Verification items for the finished model (mm, model axes). A direction names the side the tool comes from. Coordinates: 2 decimals unless noted, no trailing zeros. Order: outer loops, then holes, each group sorted by start corner. A loop starts at its lowest first (then second) coordinate and runs counter-clockwise, first axis right, second up.
Q1. Draft check along Z on faces 1 (the flat face through (7, -1, 21)), 2 (the flat face through (3, -6, 34)), 3 (the flat face through (3, -2, 27)). Enter one of: pulls with the +Z half, pulls with the -Z half, needs draft (parallel to the pull), parting line crosses it, or undercut.
Q2. Set-up check for faces 4 (the flat face through (3, -4.8, 3)), 5 (the flat face through (1.9, -2, 11.3)), 6 (the flat face through (3, -10.5, 27)): record each of +Z, -Z, +X, -X, +Y, -Y from which the full face is reachable in a straight line by a thin tool's end or side.
Q3. Thickness scan on line 1 (Z direction, x = 6, y = -8.75); line 2 (Y direction, x = 2.5, z = 25); line 3 (Y direction, x = 1, z = 5.5). Record the ranges inside material, lowest first.
Q4. Cross-section at A-A, the plane z = 10. Record the boundary of the cut face in (x, y), and give its area (3 significant figures).
Q5. Cross-section at D-D, the plane x = 6.25. Record the boundary of the cut face in (y, z), and give its area (3 significant figures).
Q6. Cross-section at B-B, the plane x = 3.5. Count the separate pieces of the cut face and the enclosed holes in it, and give its area (3 significant figures).
Q7. Depth check by flat-ended pin: P1, Ø0.7, axis at x = 5, z = 17, coming from the -Y side; P2, Ø0.7, axis at x = 3.5, y = -3, coming from the -Z side; P3, Ø2, axis at x = 6, z = 6, coming from the -Y side. Enter the tip coordinate at first touch or a pass-through.
Q8. Cross-section at C-C, the plane y = -8.75. Record the boundary of the cut face in (x, z).
from build123d import *

# Parameters (mm, degrees)
F0_W     = 7
F0_H     = 20
F0_R     = 1.75
F1_DEPTH = 2
F3_DEPTH = 2.8
F4_R     = 0.5
F5_R     = 0.5
F6_W     = 8.5
F6_H     = 8.979
F7_DEPTH = 7
F8_R     = 2.5
F9_R     = 1


with BuildPart() as f1:
    # F0 (on Front) → F1 (new body)
    with BuildSketch(Plane.XZ):
        with Locations((3.5, 10)):
            Rectangle(F0_W, F0_H)
        with Locations((3.5, 10)):
            Circle(F0_R, mode=Mode.SUBTRACT)
    extrude(amount=F1_DEPTH)

    # F2 (on face) → F3 (join)
    with BuildSketch(Plane.XZ.offset(2)):
        Polygon((7, 4.45), (3.5, 4.45), (0, 4.45), (0, 2.05), (7, 2.05), align=None)
        Polygon((0, 15.55), (3.5, 15.55), (7, 15.55), (7, 17.95), (0, 17.95), align=None)
    extrude(amount=F3_DEPTH)

    # F4
    f4_edges = [f1.edges().sort_by_distance(p)[0] for p in [
        (3.5, -4.8, 2.05),
        (3.5, -4.8, 4.45),
        (3.5, -4.8, 15.55),
        (3.5, -4.8, 17.95),
    ]]
    fillet(f4_edges, radius=F4_R)

    # F5
    f5_edges = [f1.edges().sort_by_distance(p)[0] for p in [
        (3.5, 0, 0),
    ]]
    fillet(f5_edges, radius=F5_R)

    # F6 (on face) → F7 (join, through all)
    with BuildSketch(Plane(origin=(0, 0, 0), x_dir=(0, -1, 0), z_dir=(-1, 0, 0))):
        Polygon((0, 20), (2, 20), (2, 22.221), (11.03, 22.221), (12.5, 22.221), (12.5, 34), (0, 34), align=None)
        with Locations((6.25, 27.5105)):
            Rectangle(F6_W, F6_H, mode=Mode.SUBTRACT)
    extrude(amount=-F7_DEPTH)

    # F8
    f8_edges = [f1.edges().sort_by_distance(p)[0] for p in [
        (3.5, -12.5, 34),
        (3.5, 0, 34),
    ]]
    fillet(f8_edges, radius=F8_R)

    # F9
    f9_edges = [f1.edges().sort_by_distance(p)[0] for p in [
        (3.5, -12.5, 22.221),
    ]]
    fillet(f9_edges, radius=F9_R)


solid = f1.part
Check values:
1. face 1: needs draft
1. face 2: pulls with the +Z half
1. face 3: undercut
2. face 4: -Z, +X, -X, -Y
2. face 5: +X, -X, -Y
2. face 6: +X, -X
3. line 1: z = 22.22 to 23.02, 32 to 34
3. line 2: y = -12.5 to -10.5, -2 to 0
3. line 3: y = -2 to 0
4. outline: (0, -2) - (1.75, -2) - (1.75, 0) - (0, 0) - close; (5.25, -2) - (7, -2) - (7, 0) - (5.25, 0) - close
4. area: 7.00 mm2
5. outline: (-12.5, 23.22) arc R1 ccw to (-11.5, 22.22) - (-2, 22.22) - (-2, 17.95) - (-4.3, 17.95) arc R0.5 ccw to (-4.8, 17.45) - (-4.8, 16.05) arc R0.5 ccw to (-4.3, 15.55) - (-2, 15.55) - (-2, 4.45) - (-4.3, 4.45) arc R0.5 ccw to (-4.8, 3.95) - (-4.8, 2.55) arc R0.5 ccw to (-4.3, 2.05) - (-2, 2.05) - (-2, 0) - (-0.5, 0) arc R0.5 ccw to (0, 0.5) - (0, 31.5) arc R2.5 ccw to (-2.5, 34) - (-10, 34) arc R2.5 ccw to (-12.5, 31.5) - close; hole (-10.5, 23.02) - (-2, 23.02) - (-2, 32) - (-10.5, 32) - close
5. area: 126 mm2
6. separate pieces: 2
6. enclosed holes: 1
6. area: 119 mm2
7. P1: stops at y = -4.8
7. P2: stops at z = 2.05
7. P3: stops at y = -2
8. outline: (0, 22.22) - (7, 22.22) - (7, 23.02) - (0, 23.02) - close; (0, 32) - (7, 32) - (7, 34) - (0, 34) - close
